Here's how the part is built. I have some questions about the finished solid (model axes, mm). A direction names the side the tool comes from. Give positions to 0.01 mm unless a question says otherwise; leave off trailing zeros. Loops run counter-clockwise (first coordinate to the right, second up) from the corner with the lowest first, then second, coordinate; pieces in that order, holes last. Notation, with made-up numbers: (46.5, 3.25) -> (80.5, 3.25) arc R21 cw to (80.5, 42.25) -> close; hole circle Ø1 at (-25.5, -15). An arc over 180 degrees is marked (long way). Answer in a Markdown table with one row per item. Add a question column.
Item 1: We'd pull the mould along X, two halves only. Please class faces 3 (the face through (-6.84, -11.22, 0)), 4 (the face through (-3.3, -14.88, -3.01)), 5 (the face through (-6.607, -29.755, 3.259)), 6 (the face through (13, 0, 6.35)): released by +X, released by -X, zero draft, split by the parting line, or undercut.
Item 2: If we section it at D-D (z = 4.5): Write out the boundary of the cut face in (x, y).
Item 3: Which directions (+Z, -Z, +X, -X, +Y, -Y) give clear straight access to the entire face, cutting with the end or side of a thin tool? Please do faces 1 (the face through (5, 15, -6.35)), 2 (the face through (21.199, 6.676, -3.005)).
Item 4: For P1, Ø4, axis at y = 9, z = -1.5, coming from the -X side; P2, Ø5.5, axis at x = 0, y = 26.35, coming from the -Z side; P3, Ø5, axis at x = -2, z = -2, coming from the -Y side; P4, Ø4, axis at x = 18, z = 0, coming from the +Y side, each with a flat end and sliding along its axis, tell me the tip position at first contact or that it passes through.
Item 5: If we section it at A-A (x = 0): Give the number of separate pieces and of enclosed holes in the cut face, then the cut area to 3 significant figures.
Item 6: If I drill on line 1 (Y direction, x = 0, z = 5); line 2 (Z direction, x = -16, y = 22); line 3 (X direction, y = 10, z = -0.25), over which ranges is the centre line in solid material (lowest first)?
Item 7: If we section it at B-B (y = 0): Write out the boundary of the cut face in (x, z) (3 decimals), then the cut area to 3 significant figures.
Item 8: If we section it at C-C (z = -3.25): Write out the boundary of the cut face in (x, y) (3 decimals), then the cut area to 3 significant figures.
```python
from build123d import *

# Parameters (mm, degrees)
F0_R     = 30.48
F0_R_2   = 12.7
F1_DEPTH = 6.35
F2_R     = 22.225
F2_R_2   = 15.24
F3_DEPTH = 6.35
F2_R_3   = 3.429
F4_DEPTH = 34.798
F5_SIZE  = 0.254


with BuildPart() as f1:
    # F0 (on Top) → F1 (new body)
    with BuildSketch(Plane.XY):
        Circle(F0_R)
        Circle(F0_R_2, mode=Mode.SUBTRACT)
    extrude(amount=F1_DEPTH)

    # F2 (on Top) → F3 (join)
    with BuildSketch(Plane.XY):
        Circle(F2_R)
        Circle(F2_R_2, mode=Mode.SUBTRACT)
    extrude(amount=-F3_DEPTH)

    # F2 (on Top) → F4 (cut)
    with BuildSketch(Plane.XY):
        with Locations((-22.821934, -13.17625)):
            Circle(F2_R_3)
        with Locations((0, 26.3525)):
            Circle(F2_R_3)
        with Locations((22.821934, -13.17625)):
            Circle(F2_R_3)
    extrude(amount=F4_DEPTH, mode=Mode.SUBTRACT)

    # F5
    f5_edges = [f1.edges().sort_by_distance(p)[0] for p in [
        (-30.48, 0, 0),
        (-22.225, 0, -6.35),
        (-15.24, 0, -6.35),
        (-12.7, 0, 0),
    ]]
    chamfer(f5_edges, length=F5_SIZE)


solid = f1.part
```
Recorded:
| question | item | result |
|---|---|---|
| 1 | face 3 | undercut |
| 1 | face 4 | undercut |
| 1 | face 5 | split by the parting line |
| 1 | face 6 | zero draft |
| 2 | outline | circle Ø60.96 at (0, 0); hole circle Ø6.86 at (-22.82, -13.18); hole circle Ø25.4 at (0, 0); hole circle Ø6.86 at (0, 26.35); hole circle Ø6.86 at (22.82, -13.18) |
| 3 | face 1 | -Z, +X, -X, +Y, -Y |
| 3 | face 2 | -Z |
| 4 | P1 | stops at x = -29.4 |
| 4 | P2 | passes through |
| 4 | P3 | stops at y = -30.47 |
| 4 | P4 | stops at y = 25.93 |
| 5 | separate pieces | 3 |
| 5 | enclosed holes | 0 |
| 5 | area | 271 mm^2 |
| 6 | line 1 | y = -30.48 to -12.7, 12.7 to 22.92, 29.78 to 30.48 |
| 6 | line 2 | z = 0 to 6.35 |
| 6 | line 3 | x = -19.85 to -11.5, 11.5 to 19.85 |
| 7 | outline | (-30.48, 0.254) -> (-30.226, 0) -> (-22.225, 0) -> (-22.225, -6.096) -> (-21.971, -6.35) -> (-15.494, -6.35) -> (-15.24, -6.096) -> (-15.24, 0) -> (-12.954, 0) -> (-12.7, 0.254) -> (-12.7, 6.35) -> (-30.48, 6.35) -> close; (12.7, 0.254) -> (12.954, 0) -> (15.24, 0) -> (15.24, -6.096) -> (15.494, -6.35) -> (21.971, -6.35) -> (22.225, -6.096) -> (22.225, 0) -> (30.226, 0) -> (30.48, 0.254) -> (30.48, 6.35) -> (12.7, 6.35) -> close |
| 7 | area | 314 mm^2 |
| 8 | outline | circle Ø44.45 at (0, 0); hole circle Ø30.48 at (0, 0) |
| 8 | area | 822 mm^2 |
